Can you work these out from the model? Positions are in its coordinate system, mm. Give positions to 0.01 mm unless a question says otherwise; leave off trailing zeros. Order: outer loops, then holes, each group sorted by start corner. A loop starts at its lowest first (then second) coordinate and runs counter-clockwise, first axis right, second up. Notation, with made-up numbers: M 15,80.25 L 52,80.25 A15 ccw 52,108.25 Z; hole C 72,47.25 d4. An arc over 180 degrees is marked long. Write each question's results on one line, items separated by ' | '.
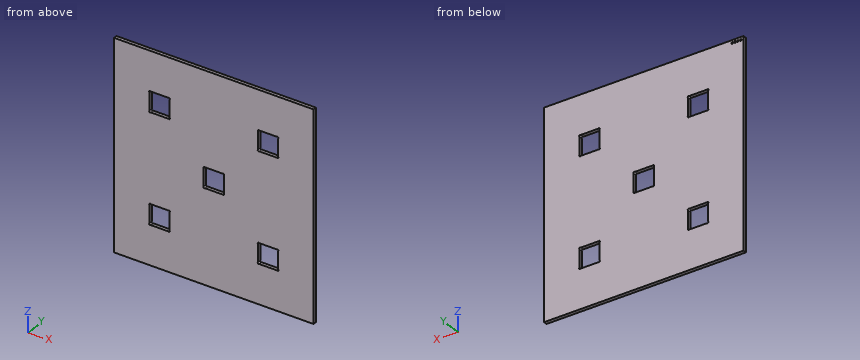
from build123d import *

# Parameters (mm, degrees)
SKETCH1_W           = 180.7718
SKETCH1_H           = 187.452
BOSS_EXTRUDE1_DEPTH = 3.175
SKETCH2_W           = 18.288
SKETCH2_H           = 18.288
CUT_EXTRUDE1_DEPTH  = 3.175
SKETCH3_R           = 0.79375
CUT_EXTRUDE2_DEPTH  = 131.246898696
SKETCH9_R           = 0.79375
CUT_EXTRUDE4_DEPTH  = 1.27
LPATTERN1_COUNT     = 4
LPATTERN1_PITCH     = 2.54


with BuildPart() as part:
    # Sketch1 → Boss-Extrude1 (new body)
    with BuildSketch(Plane(origin=(0, 0, 0), x_dir=(1, 0, 0), z_dir=(0, 1, 0))):
        Rectangle(SKETCH1_W, SKETCH1_H)
    extrude(amount=BOSS_EXTRUDE1_DEPTH)

    # Sketch2 → Cut-Extrude1 (cut)
    with BuildSketch(Plane(origin=(0, 3.175, 0), x_dir=(1, 0, 0), z_dir=(0, 1, 0))):
        Rectangle(SKETCH2_W, SKETCH2_H)
    cut_extrude1 = extrude(amount=-CUT_EXTRUDE1_DEPTH, mode=Mode.SUBTRACT)

    # Sketch3 → Cut-Extrude2 (cut, through all)
    with BuildSketch(Plane(origin=(0, 3.175, 0), x_dir=(1, 0, 0), z_dir=(0, 1, 0))):
        with Locations((8.582733992, -8.582733992)):
            Circle(SKETCH3_R)
        with Locations((-8.582733992, -8.582733992)):
            Circle(SKETCH3_R)
        with Locations((-8.582733992, 8.582733992)):
            Circle(SKETCH3_R)
        with Locations((8.582733992, 8.582733992)):
            Circle(SKETCH3_R)
    cut_extrude2 = extrude(amount=-CUT_EXTRUDE2_DEPTH, mode=Mode.SUBTRACT)

    # Sketch-Pattern1: Cut-Extrude1, Cut-Extrude2 at 4 more places
    with Locations((-49.2125, 0, 49.2125), (-49.2125, 0, -49.2125), (49.2125, 0, -49.2125), (49.2125, 0, 49.2125)):
        add(cut_extrude1, mode=Mode.SUBTRACT)
        add(cut_extrude2, mode=Mode.SUBTRACT)

    # Sketch9 → Cut-Extrude4 (cut)
    with BuildSketch(Plane(origin=(0, 3.175, 0), x_dir=(1, 0, 0), z_dir=(0, 1, 0))):
        with Locations(Location((-87.8459, -91.186, 0), (0, 0, 270))):
            Circle(SKETCH9_R)
    cut_extrude4 = extrude(amount=-CUT_EXTRUDE4_DEPTH, mode=Mode.SUBTRACT)

    # LPattern1: Cut-Extrude4 ×4
    with Locations(*[(i * LPATTERN1_PITCH, 0, 0) for i in range(1, LPATTERN1_COUNT)]):
        add(cut_extrude4, mode=Mode.SUBTRACT)


solid = part.part
(1) Imagine slicing it at A-A, the plane z = 48. Write out the boundary of the cut face in (x, y) (1 decimal), plus the area to 3 significant figures.
Data:
outline: M -90.4,0 L -58.4,0 L -58.4,3.2 L -90.4,3.2 Z; M -40.1,0 L 40.1,0 L 40.1,3.2 L -40.1,3.2 Z; M 58.4,0 L 90.4,0 L 90.4,3.2 L 58.4,3.2 Z | area: 458 mm2
(2) I need wall thicknesses on L1, parallel to Z at x = 52.5, y = 1.45; L2, parallel to X at y = 1.2, z = 47; L3, parallel to Z at x = 1, y = 2.1. Which ranges of each line are inside material? Lowest first, please. Write a range as from..to.
Data:
L1: z = -93.73..-58.36, -40.07..40.07, 58.36..93.73 | L2: x = -90.39..-58.36, -40.07..40.07, 58.36..90.39 | L3: z = -93.73..-9.14, 9.14..93.73
(3) Imagine slicing it at B-B, the plane y = 0.8. Count the separate pieces of the cut face and the enclosed holes in it, plus the area to 3 significant figures.
Data:
separate pieces: 1 | enclosed holes: 5 | area: 32,200 mm2
